Design review of the part built by this model. Coordinates are the model's own, in mm. Face numbers are marked on the shaded views. A direction names the side the tool comes from. Round coordinates to 2 decimals unless told otherwise and drop trailing zeros. Write each loop counter-clockwise with the first axis right and the second up, starting at its lowest first coordinate (ties: lowest second). Pieces come first, ordered by that corner, then holes.
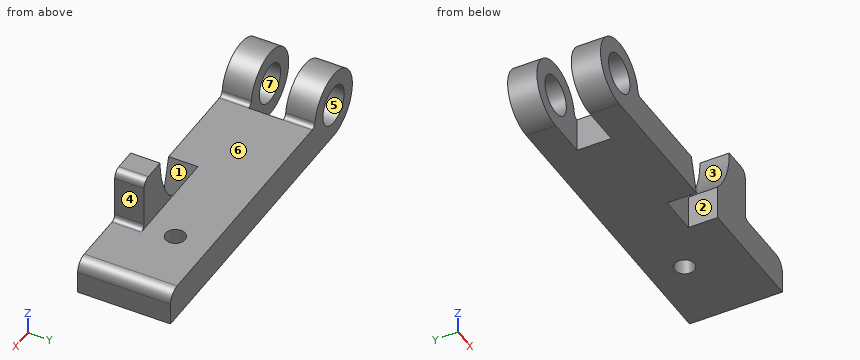
from build123d import *

# Parameters (mm, degrees)
F0_R     = 12.7
F1_DEPTH = 30.1625
F2_DEPTH = 11.1633
F4_DEPTH = 19.05
F5_DEPTH = 19.05
F6_R     = 6.35
F7_DEPTH = 22.353


with BuildPart() as f1:
    # F0 (on Front) → F1 (new body, symmetric)
    with BuildSketch(Plane.XZ):
        with BuildLine():
            ThreePointArc((25.440608, 0), (23.261179, 0.821417), (22.166074, 2.87699))
            ThreePointArc((22.166074, 2.87699), (-16.791641, 14.753058), (0, -22.352))
            Line((0, -22.352), (25.440608, -22.352))
            Line((25.440608, -22.352), (25.440608, 0))
        make_face()
        Circle(F0_R, mode=Mode.SUBTRACT)
        with BuildLine():
            Line((131.0386, 0), (117.2464, 0))
            Line((117.2464, 0), (117.2464, -22.352))
            Line((117.2464, -22.352), (194.2084, -22.352))
            Line((194.2084, -22.352), (194.2084, -7.874))
            ThreePointArc((194.2084, -7.874), (191.902159, -2.306241), (186.3344, 0))
            Line((186.3344, 0), (153.3906, 0))
            Line((153.3906, 0), (131.0386, 0))
        make_face()
        Polygon((117.2464, 0), (85.852, 0), (91.8464, -22.352), (117.2464, -22.352), align=None)
        Polygon((85.852, 0), (25.440608, 0), (25.440608, -22.352), (91.8464, -22.352), align=None)
    extrude(amount=F1_DEPTH, both=True)

    # F0 (on Front) → F2 (cut, symmetric)
    with BuildSketch(Plane.XZ):
        with BuildLine():
            ThreePointArc((25.440608, 0), (23.261179, 0.821417), (22.166074, 2.87699))
            ThreePointArc((22.166074, 2.87699), (-16.791641, 14.753058), (0, -22.352))
            Line((0, -22.352), (25.440608, -22.352))
            Line((25.440608, -22.352), (25.440608, 0))
        make_face()
        Circle(F0_R, mode=Mode.SUBTRACT)
    extrude(amount=F2_DEPTH, both=True, mode=Mode.SUBTRACT)

    # F3 (on face) → F4 (join)
    with BuildSketch(Plane.XZ.offset(30.1625)):
        Polygon((117.2464, -22.352), (117.2464, 0), (85.852, 0), (91.8464, -22.352), align=None)
        with BuildLine():
            Line((150.0886, 3.302), (150.0886, 29.720327))
            ThreePointArc((150.0886, 29.720327), (148.600702, 33.312429), (145.0086, 34.800327))
            Line((145.0086, 34.800327), (131.0386, 34.800327))
            ThreePointArc((131.0386, 34.800327), (127.464844, 16.083439), (117.2464, 0))
            Line((117.2464, 0), (131.0386, 0))
            Line((131.0386, 0), (153.3906, 0))
            ThreePointArc((153.3906, 0), (151.055733, 0.967133), (150.0886, 3.302))
        make_face()
    extrude(amount=-F4_DEPTH)

    # F3 (on face) → F5 (cut)
    with BuildSketch(Plane.XZ.offset(30.1625)):
        Polygon((117.2464, -22.352), (117.2464, 0), (85.852, 0), (91.8464, -22.352), align=None)
    extrude(amount=-F5_DEPTH, mode=Mode.SUBTRACT)

    # F6 (on face) → F7 (cut, through all)
    with BuildSketch(Plane.XY):
        with Locations((147.4724, 7.8105)):
            Circle(F6_R)
    extrude(amount=-F7_DEPTH, mode=Mode.SUBTRACT)


solid = f1.part
1) Add section D-D on y = -1.5. State the section outline as (x, z) points.
2) The part is to be moulded in two halves that separate along Z. For the marked faces 4, 5, 6 and 7, say which applies: pulls with the +Z half, pulls with the -Z half, needs draft (parallel to the pull), parting line crosses it, or undercut.
3) For line 1 along Z through (x, y) = (74.5, 14); line 2 along Y through (x, z) = (12, -15.5); line 3 along X through (y, z) = (13, -8), list the stretches that pass through material, from the lowest coordinate up.
4) Add section A-A on y = 24. State the section outline as (x, z) points, and give its area (3 significant figures).
5) For the marked faces 1, 2 and 3, list the 3-axis set-ups (+Z, -Z, +X, -X, +Y, -Y) from which the entire face can be reached by the end or side of a thin tool; tool diameter is ignored.
6) For P1, Ø9.5, axis at y = -20, z = -8.5, coming from the -X side; P2, Ø10.5, axis at x = 139.5, z = 18, coming from the +Y side; P3, Ø20.5, axis at x = 147.47, y = 7.81, coming from the +Z side, all flat-tipped, find the tip position at first contact; note any pin that passes through.
7) Add section C-C on x = 89. State the section outline as (y, z) points, and give its area (3 significant figures).
8) Add section B-B on z = 10.5. State the section outline as (x, y) points.
Computed:
1. outline: (25.44, -22.35) - (194.21, -22.35) - (194.21, -7.87) arc R7.87 ccw to (186.33, 0) - (25.44, 0) - close
2. face 4: needs draft
2. face 5: undercut
2. face 6: pulls with the +Z half
2. face 7: undercut
3. line 1: z = -22.35 to 0
3. line 2: y = -30.16 to -11.16, 11.16 to 30.16
3. line 3: x = -20.87 to -9.86, 9.86 to 143.81, 151.13 to 194.21
4. outline: (0, -22.35) - (194.21, -22.35) - (194.21, -7.87) arc R7.87 ccw to (186.33, 0) - (25.44, 0) arc R3.3 cw to (22.17, 2.88) arc R22.35 ccw (long way) to start; hole circle Ø25.4 at (0, 0)
4. area: 5,000 mm2
5. face 1: +Z, -Y
5. face 2: +Z, -Z, -Y
5. face 3: +Z, +Y, -Y
6. P1: stops at x = -22.04
6. P2: stops at y = -11.11
6. P3: stops at z = 0
7. outline: (-30.16, -22.35) - (30.16, -22.35) - (30.16, 0) - (-11.11, 0) - (-11.11, -11.74) - (-30.16, -11.74) - close
7. area: 1,120 mm2
8. outline: (-19.73, -30.16) - (-7.14, -30.16) - (-7.14, -11.16) - (-19.73, -11.16) - close; (-19.73, 11.16) - (-7.14, 11.16) - (-7.14, 30.16) - (-19.73, 30.16) - close; (7.14, -30.16) - (19.73, -30.16) - (19.73, -11.16) - (7.14, -11.16) - close; (7.14, 11.16) - (19.73, 11.16) - (19.73, 30.16) - (7.14, 30.16) - close; (124.85, -30.16) - (150.09, -30.16) - (150.09, -11.11) - (124.85, -11.11) - close
